Model file for the job. Use its own axes, mm. Face numbers are marked on the shaded views. Coordinates: 2 decimals unless noted, no trailing zeros. Loops run counter-clockwise (first coordinate to the right, second up) from the corner with the lowest first, then second, coordinate; pieces in that order, holes last. Notation, with made-up numbers: (35, 55) -> (55, 55) arc R27 cw to (55, 88) -> close; hole circle Ø10 at (62, 68.5). An arc over 180 degrees is marked (long way). Use one line per item in the form item = value.
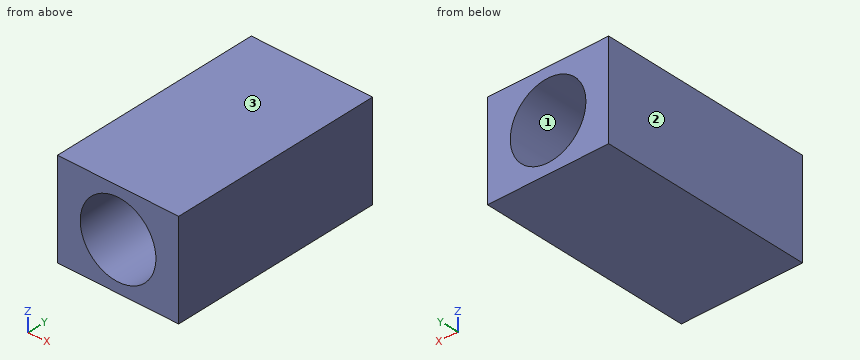
```python
from build123d import *

# Parameters (mm, degrees)
SKETCH1_W                    = 8.491382686
SKETCH1_H                    = 6.732196236
SKETCH1_R                    = 2.5
BOSS_EXTRUDE1_DEPTH          = 15
TALADRO_DE_MARGEN_PARA_M51_D = 5.3


with BuildPart() as part:
    # Sketch1 → Boss-Extrude1 (new body)
    with BuildSketch(Plane(origin=(0, 0, 0), x_dir=(1, 0, 0), z_dir=(0, 1, 0))):
        Rectangle(SKETCH1_W, SKETCH1_H)
        with Locations(Location((0, 0, 0), (0, 0, 270))):
            Circle(SKETCH1_R, mode=Mode.SUBTRACT)
    extrude(amount=BOSS_EXTRUDE1_DEPTH)

    # Taladro de margen para M51 (through all)
    with Locations(Plane(origin=(0, 15, 0), x_dir=(1, 0, 0), z_dir=(0, 1, 0))):
        with Locations((0, 0)):
            Hole(TALADRO_DE_MARGEN_PARA_M51_D / 2)


solid = part.part
```
Q1. Wall check: line 1 along Z through (x, y) = (0, 10.5); line 2 along X through (y, z) = (8.75, 0.5); line 3 along Z through (x, y) = (-0.75, 9.25). Give the ranges that are in metal, low to high.
Result:
line_1 = -3.37 to -2.65, 2.65 to 3.37
line_2 = -4.25 to -2.6, 2.6 to 4.25
line_3 = -3.37 to -2.54, 2.54 to 3.37
Q2. Band-saw the part on C-C, the plane y = 6.25. Write the cut outline in (x, z), and give its area (3 significant figures).
Result:
outline = (-4.25, -3.37) -> (4.25, -3.37) -> (4.25, 3.37) -> (-4.25, 3.37) -> close; hole circle Ø5.3 at (0, 0)
area = 35.1 mm2
Q3. Mould opens along Z. For the marked faces 1, 2 and 3 say: released by +Z, released by -Z, zero draft, split by the parting line, or undercut.
Result:
face_1 = undercut
face_2 = zero draft
face_3 = released by +Z
Q4. Band-saw the part on A-A, the plane x = -2.25. Write the cut outline in (y, z), and give its area (3 significant figures).
Result:
outline = (0, -3.37) -> (15, -3.37) -> (15, -1.4) -> (0, -1.4) -> close; (0, 1.4) -> (15, 1.4) -> (15, 3.37) -> (0, 3.37) -> close
area = 59.0 mm2
Q5. Band-saw the part on B-B, the plane z = 0. Write the cut outline in (x, y), and give its area (3 significant figures).
Result:
outline = (-4.25, 0) -> (-2.65, 0) -> (-2.65, 15) -> (-4.25, 15) -> close; (2.65, 0) -> (4.25, 0) -> (4.25, 15) -> (2.65, 15) -> close
area = 47.9 mm2
